```python
from build123d import *

# Parameters (mm, degrees)
SKETCH1_R           = 10
BOSS_EXTRUDE1_DEPTH = 6.2
CUT_EXTRUDE1_DEPTH  = 1


with BuildPart() as part:
    # Sketch1 → Boss-Extrude1 (new body)
    with BuildSketch(Plane(origin=(0, 0, 0), x_dir=(1, 0, 0), z_dir=(0, 1, 0))):
        Polygon((0, 45.002), (0, 0), (165.002, 0), (165.002, 6.2), (169.116, 6.2), (169.116, 0), (173.23, 0), (173.23, 6.2), (177.344, 6.2), (177.344, 0), (181.458, 0), (181.458, 6.2), (185.572, 6.2), (185.572, 0), (189.686, 0), (189.686, 6.2), (193.8, 6.2), (193.8, 10.314), (200, 10.314), (200, 14.428), (193.8, 14.428), (193.8, 18.542), (200, 18.542), (200, 22.656), (193.8, 22.656), (193.8, 26.77), (200, 26.77), (200, 30.884), (193.8, 30.884), (193.8, 34.998), (200, 34.998), (200, 45.002), (193.8, 45.002), (193.8, 49.116), (200, 49.116), (200, 53.23), (193.8, 53.23), (193.8, 57.344), (200, 57.344), (200, 61.458), (193.8, 61.458), (193.8, 65.572), (200, 65.572), (200, 69.686), (193.8, 69.686), (193.8, 73.8), (189.686, 73.8), (189.686, 80), (185.576, 80), (185.576, 73.8), (181.462, 73.8), (181.462, 80), (177.348, 80), (177.348, 73.8), (173.234, 73.8), (173.234, 80), (169.12, 80), (169.12, 73.8), (165.006, 73.8), (165.006, 80), (34.998, 80), (34.998, 73.8), (30.884, 73.8), (30.884, 80), (26.77, 80), (26.77, 73.8), (22.656, 73.8), (22.656, 80), (18.542, 80), (18.542, 73.8), (14.428, 73.8), (14.428, 80), (10.314, 80), (10.314, 73.8), (6.2, 73.8), (6.2, 69.686), (0, 69.686), (0, 65.572), (6.2, 65.572), (6.2, 61.458), (0, 61.458), (0, 57.344), (6.2, 57.344), (6.2, 53.23), (0, 53.23), (0, 49.116), (6.2, 49.116), (6.2, 45.002), align=None)
        with Locations((41.81119745, 37.836428286)):
            Circle(SKETCH1_R, mode=Mode.SUBTRACT)
    extrude(amount=BOSS_EXTRUDE1_DEPTH)

    # Sketch2 → Cut-Extrude1 (cut)
    with BuildSketch(Plane(origin=(0, 6.2, 0), x_dir=(1, 0, 0), z_dir=(0, 1, 0))):
        with BuildLine():
            Line((49.75994289, 65.855432978), (49.75994289, 65.529791952))
            Line((49.75994289, 65.529791952), (48.679984958, 65.529791952))
            Line((48.679984958, 65.529791952), (48.508896216, 64.694700807))
            add(Edge.make_bspline(
                [(48.508896216, 64.694700807), (48.542511188, 64.703981125), (48.607634879, 64.721960273), (48.70375561, 64.74192265), (48.795007109, 64.753956303), (48.854221195, 64.755599421), (48.882874581, 64.756394517)],
                knots=[0, 0, 0, 0, 0.000104595, 0.000202637, 0.000294305, 0.000380252, 0.000380252, 0.000380252, 0.000380252], degree=3))
            add(Edge.make_bspline(
                [(48.882874581, 64.756394517), (48.918329116, 64.755627132), (48.988041591, 64.754118262), (49.090039779, 64.739629513), (49.187406046, 64.716824019), (49.279936768, 64.684964689), (49.367803124, 64.644225145), (49.450196698, 64.593334485), (49.528354233, 64.533886392), (49.600873586, 64.465537702), (49.666663495, 64.39031595), (49.724508357, 64.309437024), (49.773641564, 64.22368693), (49.813157391, 64.132246378), (49.844711752, 64.036126289), (49.865713918, 63.934315303), (49.879699076, 63.82777308), (49.881261526, 63.754925363), (49.882058275, 63.71777773)],
                knots=[0, 0, 0, 0, 0.000106308, 0.000209029, 0.000308378, 0.000405929, 0.000502102, 0.000598312, 0.00069588, 0.000796219, 0.000896736, 0.000995218, 0.001094066, 0.001192613, 0.001293582, 0.001396995, 0.001504047, 0.001615439, 0.001615439, 0.001615439, 0.001615439], degree=3))
            add(Edge.make_bspline(
                [(49.882058275, 63.71777773), (49.881454957, 63.691904001), (49.880256474, 63.640506205), (49.874161755, 63.564175395), (49.862427212, 63.489460539), (49.846672205, 63.416351726), (49.826223012, 63.344987367), (49.801467942, 63.275163196), (49.771172974, 63.207313802), (49.737943083, 63.140797194), (49.700526636, 63.07711712), (49.65899899, 63.01756411), (49.61512458, 62.961244798), (49.567915609, 62.908763197), (49.516933277, 62.860464174), (49.462795022, 62.81606109), (49.405932841, 62.774803026), (49.345467014, 62.738364735), (49.282744904, 62.704834053), (49.216860736, 62.677326273), (49.149314243, 62.652733151), (49.079133249, 62.633130222), (49.006476719, 62.617769976), (48.931224887, 62.607337289), (48.853772422, 62.599738663), (48.801271518, 62.599262997), (48.774751584, 62.599022722)],
                knots=[0, 0, 0, 0, 7.7636e-05, 0.000154223, 0.000229512, 0.000304362, 0.000378447, 0.000452077, 0.000526407, 0.000601214, 0.00067506, 0.000747747, 0.00081887, 0.000889121, 0.000959302, 0.001029336, 0.001099058, 0.00116985, 0.001240974, 0.00131221, 0.00138383, 0.001456517, 0.001530612, 0.001606437, 0.001684346, 0.001763871, 0.001763871, 0.001763871, 0.001763871], degree=3))
            add(Edge.make_bspline(
                [(48.774751584, 62.599022722), (48.74311572, 62.59964941), (48.680875895, 62.600882346), (48.589689381, 62.613780544), (48.501955417, 62.632253525), (48.418380254, 62.660044998), (48.338214893, 62.694867759), (48.262538571, 62.738878857), (48.189417617, 62.788752758), (48.121824555, 62.847608507), (48.059090081, 62.911939162), (48.002932033, 62.981750736), (47.952918003, 63.055891016), (47.909848904, 63.134720055), (47.873111413, 63.218030723), (47.844250674, 63.306135159), (47.820956738, 63.39857302), (47.811102063, 63.462212276), (47.806096737, 63.494535542)],
                knots=[0, 0, 0, 0, 9.4843e-05, 0.000186593, 0.000275792, 0.000363484, 0.000450342, 0.000537514, 0.000625728, 0.000715478, 0.000805885, 0.000894984, 0.00098389, 0.001073836, 0.001164117, 0.001256635, 0.001351658, 0.001449737, 0.001449737, 0.001449737, 0.001449737], degree=3))
            Line((47.806096737, 63.494535542), (48.091032634, 63.494535542))
            add(Edge.make_bspline(
                [(48.091032634, 63.494535542), (48.09804354, 63.464258332), (48.11151889, 63.406063852), (48.141096962, 63.32430185), (48.177261006, 63.25144084), (48.220263522, 63.186517003), (48.271562478, 63.129903127), (48.330099889, 63.079450507), (48.395729609, 63.033934497), (48.468657753, 62.995995272), (48.545595332, 62.963638617), (48.626119873, 62.942092437), (48.708038815, 62.926942341), (48.763445623, 62.925425815), (48.791288043, 62.924663747)],
                knots=[0, 0, 0, 0, 9.3172e-05, 0.000179081, 0.000260145, 0.000336703, 0.000411917, 0.000488562, 0.000568128, 0.000650923, 0.00073478, 0.000817953, 0.000900557, 0.000983994, 0.000983994, 0.000983994, 0.000983994], degree=3))
            add(Edge.make_bspline(
                [(48.791288043, 62.924663747), (48.818464632, 62.92540831), (48.871975557, 62.92687436), (48.950725887, 62.938158321), (49.026756137, 62.955536975), (49.099316096, 62.981544629), (49.169675493, 63.013153767), (49.236054556, 63.053716729), (49.300373595, 63.100398317), (49.360633401, 63.153880403), (49.415823473, 63.212817197), (49.464587955, 63.275843118), (49.505207012, 63.343077686), (49.539437239, 63.413356903), (49.565429874, 63.487451023), (49.583972765, 63.565012803), (49.594861254, 63.646233821), (49.59635911, 63.701632409), (49.597122378, 63.729862065)],
                knots=[0, 0, 0, 0, 8.15e-05, 0.000160473, 0.000238226, 0.000315066, 0.000391338, 0.000469218, 0.000547964, 0.000629516, 0.000710512, 0.000789892, 0.000868102, 0.000945761, 0.001024012, 0.00110315, 0.001184644, 0.001269321, 0.001269321, 0.001269321, 0.001269321], degree=3))
            add(Edge.make_bspline(
                [(49.597122378, 63.729862065), (49.596525043, 63.755330782), (49.595355845, 63.805182173), (49.585803113, 63.878115739), (49.569187002, 63.947124856), (49.546123911, 64.012542768), (49.516841786, 64.074431176), (49.481058346, 64.132853952), (49.438102049, 64.187041073), (49.389032979, 64.237017889), (49.33527747, 64.283141454), (49.275910647, 64.322460733), (49.212174856, 64.355538715), (49.144838005, 64.384084685), (49.072298418, 64.40458679), (48.995992616, 64.419979086), (48.915096602, 64.428883022), (48.859787478, 64.430118449), (48.831357153, 64.430753491)],
                knots=[0, 0, 0, 0, 7.6388e-05, 0.000149519, 0.000220172, 0.000288967, 0.000357247, 0.000425206, 0.000494043, 0.000564207, 0.000635056, 0.000706145, 0.000777268, 0.000850264, 0.000925136, 0.001002969, 0.001083601, 0.001168886, 0.001168886, 0.001168886, 0.001168886], degree=3))
            add(Edge.make_bspline(
                [(48.831357153, 64.430753491), (48.806747339, 64.430226812), (48.755934317, 64.429139353), (48.677990038, 64.421132459), (48.596082547, 64.408215385), (48.510525826, 64.390447861), (48.421062936, 64.367196813), (48.327882673, 64.339334373), (48.230789117, 64.306022274), (48.165368038, 64.280865194), (48.131737762, 64.267932978)],
                knots=[0, 0, 0, 0, 7.3822e-05, 0.000152423, 0.000234822, 0.000322511, 0.00041445, 0.000512043, 0.000614219, 0.000722306, 0.000722306, 0.000722306, 0.000722306], degree=3))
            Line((48.131737762, 64.267932978), (48.457378788, 65.855432978))
            Line((48.457378788, 65.855432978), (49.75994289, 65.855432978))
        make_face()
        Polygon((51.940847338, 65.936843234), (51.998724942, 65.936843234), (51.998724942, 63.738766311), (52.365071096, 63.738766311), (52.365071096, 63.413125286), (51.998724942, 63.413125286), (51.998724942, 62.680432978), (51.713789044, 62.680432978), (51.713789044, 63.413125286), (50.207699301, 63.413125286), align=None)
        Polygon((51.713789044, 63.738766311), (51.713789044, 65.117652529), (50.767394814, 63.738766311), align=None, mode=Mode.SUBTRACT)
    extrude(amount=-CUT_EXTRUDE1_DEPTH, mode=Mode.SUBTRACT)


solid = part.part
```
Geometry check sheet. Reference: the model listing, model coordinates, mm. A direction names the side the tool comes from. Give positions to 0.01 mm unless a question says otherwise; leave off trailing zeros. Order: outer loops, then holes, each group sorted by start corner. A loop starts at its lowest first (then second) coordinate and runs counter-clockwise, first axis right, second up.
1. Section check A-A, the plane x = 37. Enter the section's corners in (y, z).
2. Access from +Z, -Z, +X, -X, +Y, -Y to the whole of each face (thin tool, end or side, straight path). Record for faces 1 (the face through (165.002, 3, -3)), 2 (the face through (197, 3, -45.002)), 3 (the face through (34.998, 3, -77)).
3. Thickness scan on L1, parallel to X at y = 4.25, z = -4; L2, parallel to X at y = 3.5, z = -38; L3, parallel to X at y = 2.5, z = -39.5. Record the ranges inside material, lowest first.
4. Release check for a two-part mould opening along X. For faces 4 (the face through (200, 3, -68)), 5 (the face through (29, 3, -80)), 6 (the face through (175, 3, -6.2)), 7 (the face through (175, 3, -73.8)) record: pulls with the +X half, pulls with the -X half, needs draft (parallel to the pull), parting line crosses it, or undercut.
5. Gauge pin test, flat ends, axial feed: pin 1 Ø3 at (y, z) = (2.5, -75.5) entering from +X; pin 2 Ø12 at (x, z) = (119, -61.5) entering from -Y; pin 3 Ø1.2 at (x, y) = (166, 3) entering from +Z; pin 4 Ø2 at (y, z) = (3, -32.5) entering from +X. Record the tip position at first contact, or that the pin passes through.
Values follow:
1. outline: (0, -80) - (6.2, -80) - (6.2, -46.6) - (0, -46.6) - close; (0, -29.07) - (6.2, -29.07) - (6.2, 0) - (0, 0) - close
2. face 1: +Z, +Y, -Y
2. face 2: +X, +Y, -Y
2. face 3: -Z, +Y, -Y
3. L1: x = 0 to 165, 169.12 to 173.23, 177.34 to 181.46, 185.57 to 189.69
3. L2: x = 0 to 31.81, 51.81 to 200
3. L3: x = 0 to 31.95, 51.67 to 200
4. face 4: pulls with the +X half
4. face 5: needs draft
4. face 6: undercut
4. face 7: undercut
5. pin 1: stops at x = 189.69
5. pin 2: stops at y = 0
5. pin 3: stops at z = -6.2
5. pin 4: stops at x = 193.8
